Can you work these out from the model? Positions are in its coordinate system, mm. Coordinates: 2 decimals unless noted, no trailing zeros. Loops run counter-clockwise (first coordinate to the right, second up) from the corner with the lowest first, then second, coordinate; pieces in that order, holes last. Notation, with made-up numbers: (8, -25.5) - (65, -25.5) arc R31 ccw to (65, 9.5) - close; hole circle Ø9 at (-39.75, 43). An arc over 180 degrees is marked (long way). Put each result on its own line as item: value. Start each with the question number.
from build123d import *

# Parameters (mm, degrees)
SKETCH2_R               = 26.9875
BOSS_EXTRUDE1_DEPTH     = 11.5951
SHELL1_T                = -1.5875
CUT_EXTRUDE1_DEPTH      = 40.456334983
CUT_EXTRUDE1_DEPTH_BACK = 40.456334983
SKETCH5_R               = 12.7
CUT_EXTRUDE2_DEPTH      = 38.1
CIRPATTERN3_COUNT       = 20
CUT_EXTRUDE3_DEPTH      = 40.456334983
CUT_EXTRUDE3_DEPTH_BACK = 40.456334983


with BuildPart() as part:
    # Sketch2 → Boss-Extrude1 (new body)
    with BuildSketch(Plane(origin=(0, 0, 0), x_dir=(1, 0, 0), z_dir=(0, 1, 0))):
        with Locations(Location((0, 0, 0), (0, 0, 270))):
            Circle(SKETCH2_R)
    extrude(amount=BOSS_EXTRUDE1_DEPTH)

    # Shell1
    shell1_openings = [part.faces().sort_by_distance(p)[0] for p in [
        (0, 11.5951, 0),
    ]]
    offset(amount=SHELL1_T, openings=shell1_openings, kind=Kind.INTERSECTION)

    # Sketch5 → Cut-Extrude1 (cut, two sides: drawn at the far end of the back side and taken through both)
    with BuildSketch(Plane(origin=(0, 1.5875, 0), x_dir=(1, 0, 0), z_dir=(0, 1, 0)).offset(-CUT_EXTRUDE1_DEPTH_BACK)):
        with Locations(Location((0, 0, 0), (0, 0, 270))):
            Circle(SKETCH5_R)
    extrude(amount=CUT_EXTRUDE1_DEPTH + CUT_EXTRUDE1_DEPTH_BACK, mode=Mode.SUBTRACT)

    # Sketch6 → Cut-Extrude2 (cut)
    with BuildSketch(Plane.XY):
        Polygon((0, 1.5875), (6.413577678, 1.5875), (0, 5.8801), (-6.413577678, 5.8801), align=None)
    cut_extrude2 = extrude(amount=-CUT_EXTRUDE2_DEPTH, mode=Mode.SUBTRACT)

    # CirPattern3: Cut-Extrude2 ×20 about axis
    cirpattern3_axis = Axis((0, 0, 0), (0, 1, 0))
    for i in range(1, CIRPATTERN3_COUNT):
        add(cut_extrude2.rotate(cirpattern3_axis, i * 360 / CIRPATTERN3_COUNT), mode=Mode.SUBTRACT)

    # Sketch7 → Cut-Extrude3 (cut, two sides: drawn at the far end of the back side and taken through both)
    with BuildSketch(Plane(origin=(0, 1.5875, 0), x_dir=(1, 0, 0), z_dir=(0, 1, 0)).offset(-CUT_EXTRUDE3_DEPTH_BACK)):
        with BuildLine():
            ThreePointArc((-23.799267157, -0.79375), (-20.913926743, -11.386080292), (-13.583355992, -19.558312715))
            Line((-13.583355992, -19.558312715), (-8.793031725, -11.261227701))
            ThreePointArc((-8.793031725, -11.261227701), (-12.661565337, -6.619472748), (-14.26543435, -0.79375))
            Line((-14.26543435, -0.79375), (-23.799267157, -0.79375))
        make_face()
        with BuildLine():
            ThreePointArc((-11.560892407, 20.81780303), (-20.318117433, 12.418102118), (-23.799267157, 0.79375))
            Line((-23.799267157, 0.79375), (-14.26543435, 0.79375))
            ThreePointArc((-14.26543435, 0.79375), (-12.064905455, 7.653150502), (-6.79728956, 12.567000871))
            Line((-6.79728956, 12.567000871), (-11.560892407, 20.81780303))
        make_face()
        with BuildLine():
            ThreePointArc((10.14631767, 21.542687715), (0, 23.8125), (-10.14631767, 21.542687715))
            Line((-10.14631767, 21.542687715), (-5.355993404, 13.245602701))
            ThreePointArc((-5.355993404, 13.245602701), (0, 14.2875), (5.355993404, 13.245602701))
            Line((5.355993404, 13.245602701), (10.14631767, 21.542687715))
        make_face()
        with BuildLine():
            ThreePointArc((6.79728956, 12.567000871), (12.064905455, 7.653150502), (14.26543435, 0.79375))
            Line((14.26543435, 0.79375), (23.799267157, 0.79375))
            ThreePointArc((23.799267157, 0.79375), (20.318117433, 12.418102118), (11.560892407, 20.81780303))
            Line((11.560892407, 20.81780303), (6.79728956, 12.567000871))
        make_face()
        with BuildLine():
            Line((8.793031725, -11.261227701), (13.583355992, -19.558312715))
            ThreePointArc((13.583355992, -19.558312715), (20.913926743, -11.386080292), (23.799267157, -0.79375))
            Line((23.799267157, -0.79375), (14.26543435, -0.79375))
            ThreePointArc((14.26543435, -0.79375), (12.661565337, -6.619472748), (8.793031725, -11.261227701))
        make_face()
        with BuildLine():
            Line((-7.484697224, -12.170125871), (-12.248300071, -20.42092803))
            ThreePointArc((-12.248300071, -20.42092803), (0, -23.8125), (12.248300071, -20.42092803))
            Line((12.248300071, -20.42092803), (7.484697224, -12.170125871))
            ThreePointArc((7.484697224, -12.170125871), (0, -14.2875), (-7.484697224, -12.170125871))
        make_face()
    extrude(amount=CUT_EXTRUDE3_DEPTH + CUT_EXTRUDE3_DEPTH_BACK, mode=Mode.SUBTRACT)


solid = part.part
Q1. Will these pins go through, and if not, where does the flat tip stop? pin 1 (1.5 mm diameter, centred on x = 15, y = 6, fed in from +Z); pin 2 (3 mm diameter, centred on x = -25, z = -3.5, fed in from -Y); pin 3 (3 mm diameter, centred on y = 4, z = -13.5, fed in from +X); pin 4 (1.3 mm diameter, centred on x = -17, y = 0.5, fed in from -Z).
Q2. Please list where these lines run through material, in increasing order: line 1 along X through (y, z) = (1.25, 0); line 2 along X through (y, z) = (9, 0); line 3 along Z through (x, y) = (13, 0.75). Write a range as [from, to].
Q3. I want a section at A-A on z = 4. Count the separate pieces of the cut face and the enclosed holes in it, and give its area (3 significant figures).
Q4. I want a section at B-B on y = 9. List the corners of the cut face in (x, z) for me (1 decimal).
Q5. We'd pull the mould along Y, two halves only. Please class faces 1 (the flat face through (-6, 0, 12)), 2 (the cylindrical face through (0.147, 0.783, -23.812)), 3 (the flat face through (-3, 5.88, -26)): released by +Y, released by -Y, zero draft, split by the parting line, or undercut.
Calculated:
1. pin 1: z = 22.92
1. pin 2: y = 0
1. pin 3: x = 24.17
1. pin 4: z = -21.47
2. line 1: [-26.99, -12.7], [12.7, 26.99]
2. line 2: [-26.99, -25.4], [25.4, 26.99]
2. line 3: [-23.65, -19.95], [-5.93, 5.93], [18.55, 23.65]
3. separate pieces: 8
3. enclosed holes: 0
3. area: 37.7 mm2
4. outline: circle Ø54 at (0, 0); hole circle Ø50.8 at (0, 0)
5. face 1: released by -Y
5. face 2: zero draft
5. face 3: undercut
